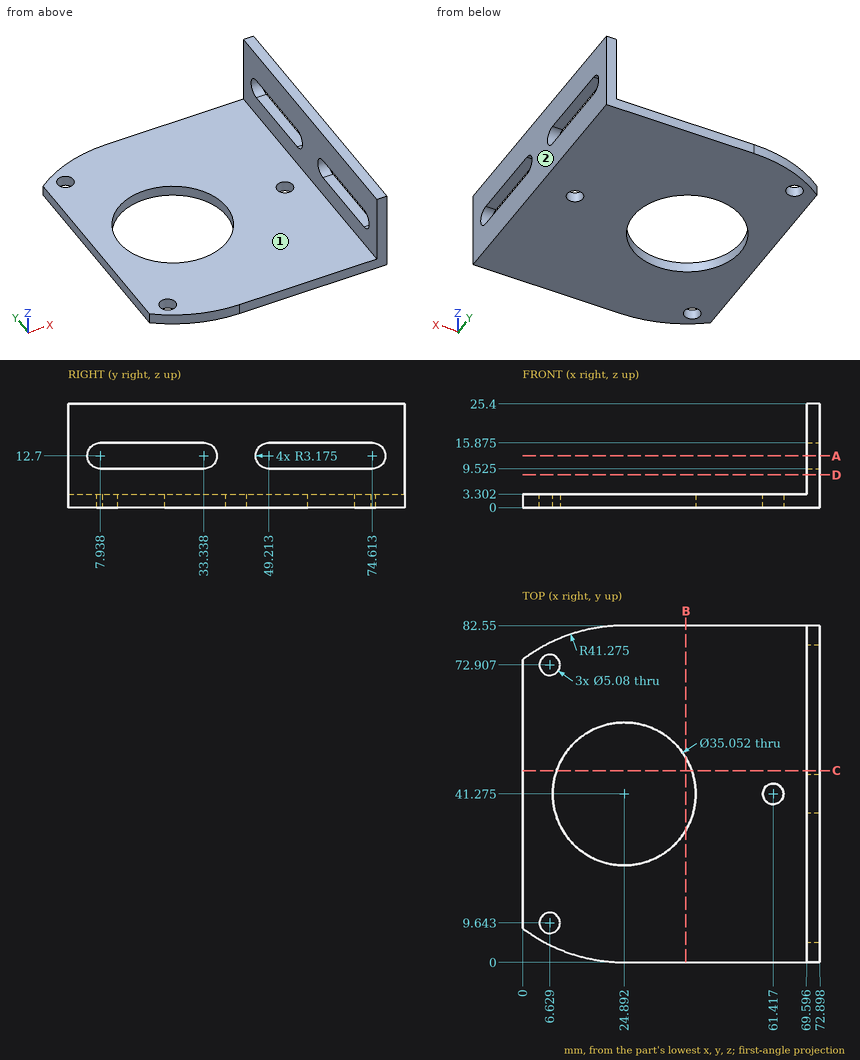
Print and shaded views of the part. All mm, measured from the part's lowest x, y and z. A direction names the side the tool comes from. Round coordinates to 2 decimals unless told otherwise and drop trailing zeros. Write each loop counter-clockwise with the first axis right and the second up, starting at its lowest first coordinate (ties: lowest second). Pieces come first, ordered by that corner, then holes. Notation, with made-up numbers: (68, 20) - (122, 20) arc R19 ccw to (122, 26) - close; hole circle Ø10 at (22.5, 58.5). An arc over 180 degrees is marked (long way). One line per item, written item: value.
(1) Cut at A-A, the plane z = 12.7. Give the cut face in (x, y).
Values follow:
outline: (69.6, 0) - (72.9, 0) - (72.9, 4.76) - (69.6, 4.76) - close; (69.6, 36.51) - (72.9, 36.51) - (72.9, 46.04) - (69.6, 46.04) - close; (69.6, 77.79) - (72.9, 77.79) - (72.9, 82.55) - (69.6, 82.55) - close
(2) Drop flat-ended pins along their axis: P1, Ø1, axis at x = 57, y = 27, coming from the +Z side; P2, Ø1.5, axis at y = 26, z = 21.5, coming from the -X side; P3, Ø10, axis at x = 59.5, z = 9.5, coming from the +Y side. Give the stop position or say it passes through.
Values follow:
P1: stops at z = 3.3
P2: stops at x = 69.6
P3: passes through
(3) 3-axis set-ups, long thin cutter, end or side, ignore diameter. For the marked faces 1 and 2: which of +Z, -Z, +X, -X, +Y, -Y reach the whole face in a straight line?
Values follow:
face 1: +Z, -X, +Y, -Y
face 2: +Z, -Z, +X, +Y, -Y
(4) Wall check: probe 1 along X at (y, z) = (19.5, 4); probe 2 along Z at (x, y) = (49, 55.5); probe 3 along X at (y, z) = (29, 2) (1 decimal). Give the ranges that are in metal, low to high.
Values follow:
probe 1: x = 69.6 to 72.9
probe 2: z = 0 to 3.3
probe 3: x = 0 to 12.4, 37.4 to 72.9
(5) Cut at D-D, the plane z = 8. Give the cut face in (x, y).
Values follow:
outline: (69.6, 0) - (72.9, 0) - (72.9, 82.55) - (69.6, 82.55) - close
(6) Cut at B-B, the plane x = 40. Give the cut face in (y, z), plus the area to 3 significant figures.
Values follow:
outline: (0, 0) - (32.39, 0) - (32.39, 3.3) - (0, 3.3) - close; (50.16, 0) - (82.55, 0) - (82.55, 3.3) - (50.16, 3.3) - close
area: 214 mm²
(7) Cut at C-C, the plane y = 47. Give the cut face in (x, z).
Values follow:
outline: (0, 0) - (8.33, 0) - (8.33, 3.3) - (0, 3.3) - close; (41.46, 0) - (72.9, 0) - (72.9, 10.42) - (69.6, 10.42) - (69.6, 3.3) - (41.46, 3.3) - close; (69.6, 14.98) - (72.9, 14.98) - (72.9, 25.4) - (69.6, 25.4) - close
